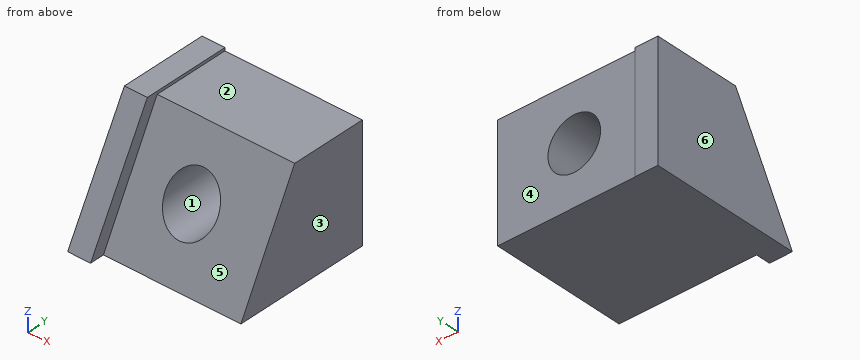
```python
from build123d import *

# Parameters (mm, degrees)
F0_W      = 152.1705836058
F0_H      = 152.1167457104
F1_DEPTH  = 127
F3_DEPTH  = 254
F4_R      = 29.1263890726
F5_DEPTH  = 2540
F7_W      = 168.390661478
F7_H      = 130.2470117807
F8_DEPTH  = 25.4
F10_DEPTH = 2540


with BuildPart() as f1:
    # F0 (on Top) → F1 (new body)
    with BuildSketch(Plane.XY):
        with Locations((0.122949481, 0.0709816813)):
            Rectangle(F0_W, F0_H)
    extrude(amount=F1_DEPTH)

    # F2 (on face) → F3 (cut)
    with BuildSketch(Plane(origin=(-75.9623423219, 0, 0), x_dir=(0, -1, 0), z_dir=(-1, 0, 0))):
        Polygon((75.9873911738, 127), (8.6493911222, 127), (75.9873911738, 0), align=None)
    extrude(amount=-F3_DEPTH, mode=Mode.SUBTRACT)

    # F4 (on face) → F5 (cut)
    with BuildSketch(Plane(origin=(0, 76.1293545365, 0), x_dir=(-1, 0, 0), z_dir=(0, 1, 0))):
        with Locations((8.6046149954, 64.465470612)):
            Circle(F4_R)
    extrude(amount=-F5_DEPTH, mode=Mode.SUBTRACT)

    # F7 (on face) → F8 (join)
    with BuildSketch(Plane(origin=(-75.9623423219, 0, 0), x_dir=(0, -1, 0), z_dir=(-1, 0, 0))):
        with Locations((7.8207552433, 65.1235058904)):
            Rectangle(F7_W, F7_H)
    extrude(amount=F8_DEPTH)

    # F9 (on face) → F10 (cut)
    with BuildSketch(Plane.YZ.offset(-75.9623423219)):
        Polygon((-92.0160859823, 0), (-20.8989176899, 130.2470117807), (-92.0160859823, 130.2470117807), align=None)
    extrude(amount=-F10_DEPTH, mode=Mode.SUBTRACT)


solid = f1.part
```
Here's how the part is built. I have some questions about the finished solid (model axes, mm). Face numbers are marked on the shaded views. A direction names the side the tool comes from. Round coordinates to 2 decimals unless told otherwise and drop trailing zeros. Loops run counter-clockwise (first coordinate to the right, second up) from the corner with the lowest first, then second, coordinate; pieces in that order, holes last.
1. Will these pins go through, and if not, where does the flat tip stop? pin 1 (3 mm diameter, centred on x = -64, z = 100, fed in from +Y); pin 2 (6 mm diameter, centred on x = -45.5, y = 12, fed in from +Z); pin 3 (1 mm diameter, centred on x = 54.5, z = 27, fed in from -Y).
Answers:
pin 1: stops at y = 76.13
pin 2: stops at z = 127
pin 3: stops at y = -61.94
2. Suppose I cut it at C-C, the plane y = -23.5. Please give me the cut outline in (x, z), and give its area (3 significant figures).
Answers:
outline: (-101.36, 0) - (76.21, 0) - (76.21, 98.99) - (-75.96, 98.99) - (-75.96, 125.48) - (-101.36, 125.48) - close; hole circle Ø58.25 at (-8.6, 64.47)
area: 15,600 mm2
3. Suppose I cut it at D-D, the plane z = 117.5. Please give me the cut outline in (x, y), and give its area (3 significant figures).
Answers:
outline: (-101.36, -27.86) - (-75.96, -27.86) - (-75.96, -13.69) - (76.21, -13.69) - (76.21, 76.13) - (-75.96, 76.13) - (-75.96, 76.37) - (-101.36, 76.37) - close
area: 16,300 mm2
4. Suppose I cut it at B-B, the plane z = 48. Please give me the cut outline in (x, y), and give its area (3 significant figures).
Answers:
outline: (-101.36, -65.81) - (-75.96, -65.81) - (-75.96, -50.54) - (-32.63, -50.54) - (-32.63, 76.13) - (-75.96, 76.13) - (-75.96, 76.37) - (-101.36, 76.37) - close; (15.42, -50.54) - (76.21, -50.54) - (76.21, 76.13) - (15.42, 76.13) - close
area: 16,800 mm2
5. For the marked faces 4, 5 and 6, which set-ups out of +Z, -Z, +X, -X, +Y, -Y let a thin tool reach every point of the face, with its end or its side?
Answers:
face 4: +Z, -Z, +X, +Y
face 5: +Z, +X, -Y
face 6: +Z, -Z, -X, +Y, -Y
6. If I drill on probe 1 along X at (y, z) = (58, 63); probe 2 along Z at (x, y) = (-59, 59); probe 3 along Z at (x, y) = (17, 21), over which ranges is the centre line in solid material (lowest first)?
Answers:
probe 1: x = -101.36 to -37.69, 20.48 to 76.21
probe 2: z = 0 to 127
probe 3: z = 0 to 50.58, 78.35 to 127
7. Thinking about a two-plate mould opening in X: for the marked faces 1, 2 and 3, which applies, released by +X, released by -X, zero draft, split by the parting line, or undercut?
Answers:
face 1: undercut
face 2: zero draft
face 3: released by +X
8. Suppose I cut it at A-A, the plane x = 3.5. Please give me the cut outline in (y, z).
Answers:
outline: (-75.99, 0) - (76.13, 0) - (76.13, 37.97) - (-55.85, 37.97) - close; (-27.76, 90.96) - (76.13, 90.96) - (76.13, 127) - (-8.65, 127) - close
